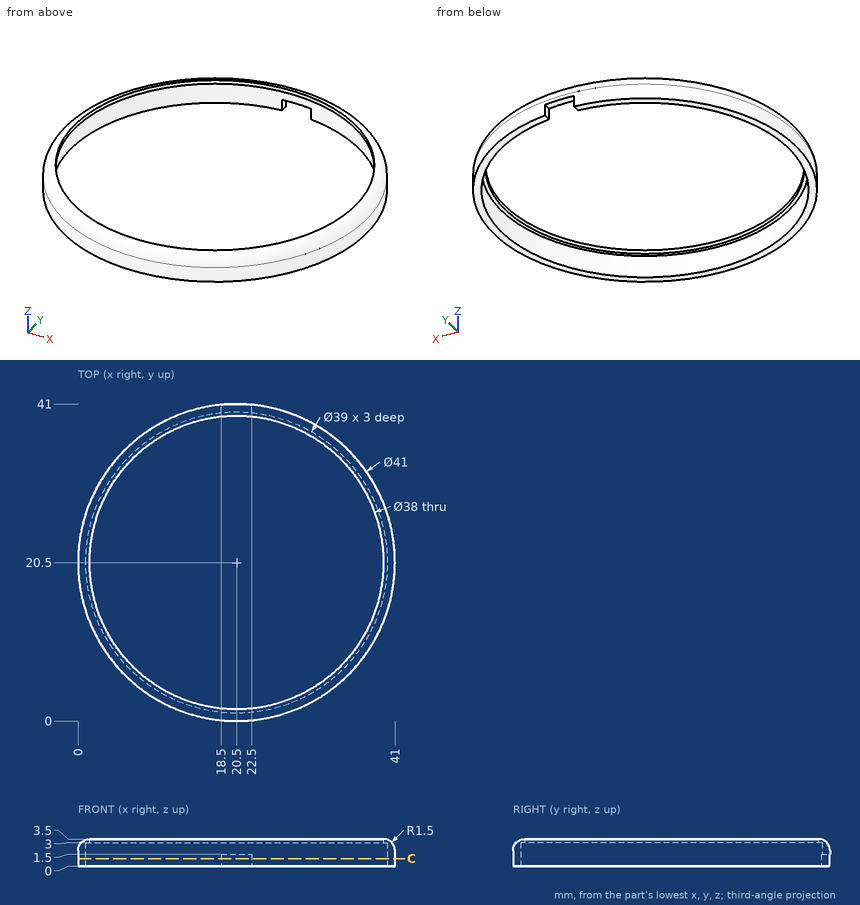
For this review, use the dimensioned drawing (mm, ordinates from the lowest corner) and the shaded views. Coordinates: 2 decimals unless noted, no trailing zeros. Order: outer loops, then holes, each group sorted by start corner. A loop starts at its lowest first (then second) coordinate and runs counter-clockwise, first axis right, second up. Notation, with made-up numbers: M 22.25,-17 L 80.25,-17 A22 ccw 80.25,19 Z; hole C 59.25,29 d3. An arc over 180 degrees is marked long. Answer as a JSON object with one key per item and string values. Group by question number.
1) For pin 1 (2 mm diameter, centred on y = 36, z = 1, fed in from -X), flat-tipped, find the tip position at first contact; note if it passes through.
2) Add section C-C, the plane z = 0.95. Write out the cut boundary in (x, y), then the cut area to 3 significant figures.
3) Wall thickness on L1, parallel to X at y = 20.5, z = 0.85; L2, parallel to Y at x = 20.5, z = 1.25: over which ranges is each line inside the solid? List them lowest first.
Computed values:
{
 "1": {"pin 1": "stops at x = 6.01"},
 "2": {"outline": "M 18.5,39.9 L 18.5,40.9 A20.5 ccw long 22.5,40.9 L 22.5,39.9 A19.5 cw long Z", "area": "122 mm^2"},
 "3": {"L1": "x = 0 to 1, 40 to 41", "L2": "y = 0 to 1"}
}
